from build123d import *

# Parameters (mm, degrees)
SKETCH2_R                   = 15.875
BOSS_EXTRUDE1_DEPTH         = 25.4
F_1_2_20_TAPPED_HOLE1_D     = 4.826
F_1_2_20_TAPPED_HOLE1_DEPTH = 31.75
F_1_2_20_TAPPED_HOLE1_TIP   = 1.449876674
F_1_2_20_TAPPED_HOLE2_D     = 4.1656
F_1_2_20_TAPPED_HOLE2_DEPTH = 31.75
F_1_2_20_TAPPED_HOLE2_TIP   = 1.251472497
F_1_2_20_TAPPED_HOLE3_D     = 4.1656
F_1_2_20_TAPPED_HOLE3_DEPTH = 31.75
F_1_2_20_TAPPED_HOLE3_TIP   = 1.251472497


with BuildPart() as part:
    # Sketch2 → Boss-Extrude1 (new body)
    with BuildSketch(Plane.XY):
        Polygon((-38.1, 60.452), (-50.8, 47.752), (-50.8, 0), (0, 0), (0, 47.752), (-12.7, 60.452), align=None)
        with Locations((-25.4, 35.052)):
            Circle(SKETCH2_R, mode=Mode.SUBTRACT)
    extrude(amount=BOSS_EXTRUDE1_DEPTH)

    # 1/2-20 Tapped Hole1
    with Locations(Plane(origin=(-25.4, 60.452, 12.7), x_dir=(1, 0, 0), z_dir=(0, 1, 0))):
        with Locations((0, 0)):
            Hole(F_1_2_20_TAPPED_HOLE1_D / 2, depth=F_1_2_20_TAPPED_HOLE1_DEPTH)
            with Locations((0, 0, -(F_1_2_20_TAPPED_HOLE1_DEPTH + F_1_2_20_TAPPED_HOLE1_TIP / 2))):  # 118° drill point
                Cone(0, F_1_2_20_TAPPED_HOLE1_D / 2, F_1_2_20_TAPPED_HOLE1_TIP, mode=Mode.SUBTRACT)

    # 1/2-20 Tapped Hole2
    with Locations(Plane(origin=(-44.924994652, 53.627005348, 12.7), x_dir=(-0.707106781187, -0.707106781187, 0), z_dir=(-0.707106781187, 0.707106781187, 0))):
        with Locations((0, 0)):
            Hole(F_1_2_20_TAPPED_HOLE2_D / 2, depth=F_1_2_20_TAPPED_HOLE2_DEPTH)
            with Locations((0, 0, -(F_1_2_20_TAPPED_HOLE2_DEPTH + F_1_2_20_TAPPED_HOLE2_TIP / 2))):  # 118° drill point
                Cone(0, F_1_2_20_TAPPED_HOLE2_D / 2, F_1_2_20_TAPPED_HOLE2_TIP, mode=Mode.SUBTRACT)

    # 1/2-20 Tapped Hole3
    with Locations(Plane(origin=(-6.824994652, 54.576994652, 12.7), x_dir=(0.707106781187, -0.707106781187, 0), z_dir=(0.707106781187, 0.707106781187, 0))):
        with Locations((0, 0)):
            Hole(F_1_2_20_TAPPED_HOLE3_D / 2, depth=F_1_2_20_TAPPED_HOLE3_DEPTH)
            with Locations((0, 0, -(F_1_2_20_TAPPED_HOLE3_DEPTH + F_1_2_20_TAPPED_HOLE3_TIP / 2))):  # 118° drill point
                Cone(0, F_1_2_20_TAPPED_HOLE3_D / 2, F_1_2_20_TAPPED_HOLE3_TIP, mode=Mode.SUBTRACT)


solid = part.part
Geometry check sheet. Reference: the model listing, model coordinates, mm. Round coordinates to 2 decimals unless told otherwise and drop trailing zeros. Write each loop counter-clockwise with the first axis right and the second up, starting at its lowest first coordinate (ties: lowest second). Pieces come first, ordered by that corner, then holes.
Item 1: Section check A-A (x = -25.4). Record the boundary of the cut face in (y, z).
Determined:
outline: (0, 0) - (19.18, 0) - (19.18, 25.4) - (0, 25.4) - close; (50.93, 0) - (60.45, 0) - (60.45, 10.29) - (50.93, 10.29) - close; (50.93, 15.11) - (60.45, 15.11) - (60.45, 25.4) - (50.93, 25.4) - close
Item 2: Section check D-D (x = -19). Record the boundary of the cut face in (y, z).
Determined:
outline: (0, 0) - (20.52, 0) - (20.52, 25.4) - (0, 25.4) - close; (49.58, 0) - (60.45, 0) - (60.45, 25.4) - (49.58, 25.4) - close
Item 3: Mould release check, pull along Y, two halves, no side actions. Record for faces 1 (the face through (-18.07, 20.97, 12.52)), 2 (the face through (-22.99, 55.53, 12.59)), 3 (the face through (-42.95, 55.6, 12.52)): +Y half, -Y half, draft (parallel to the pull), parting line (faces both ways), or undercut.
Determined:
face 1: undercut
face 2: draft
face 3: +Y half
Item 4: Section check C-C (z = 12.7). Record the boundary of the cut face in (x, y) (3 decimals), plus the area to 3 significant figures.
Determined:
outline: (-50.8, 0) - (0, 0) - (0, 47.752) - (-5.352, 53.104) - (-13.221, 45.235) arc R15.875 cw (long way) to (-38.403, 44.159) - (-46.398, 52.154) - (-50.8, 47.752) - close; (-43.452, 55.1) - (-35.583, 47.231) arc R15.875 cw to (-27.813, 50.743) - (-27.813, 60.452) - (-38.1, 60.452) - close; (-22.987, 50.743) arc R15.875 cw to (-16.293, 48.055) - (-8.298, 56.05) - (-12.7, 60.452) - (-22.987, 60.452) - close
area: 1,980 mm2
Item 5: Material ranges on line 1 along Y through (x, z) = (-25, 5.5); line 2 along Y through (x, z) = (-3, 10.5); line 3 along Y through (x, z) = (-15, 12), recorded low to high.
Determined:
line 1: y = 0 to 19.18, 50.92 to 60.45
line 2: y = 0 to 50.75
line 3: y = 0 to 23.06, 49.18 to 60.45
Item 6: Go/stop test with flat-tipped pins: pin 1 Ø5 at (x, z) = (-41, 19) entering from +Y; pin 2 Ø4.5 at (x, z) = (-25.4, 12.7) entering from +Y. Record where each tip stops, or that it passes through.
Determined:
pin 1: stops at y = 60.05
pin 2: stops at y = 19.34
Item 7: Section check B-B (y = 30.5). Record the boundary of the cut face in (x, z).
Determined:
outline: (-50.8, 0) - (-40.61, 0) - (-40.61, 25.4) - (-50.8, 25.4) - close; (-10.19, 0) - (0, 0) - (0, 25.4) - (-10.19, 25.4) - close
